Geometry check sheet. Reference: the model listing, model coordinates, mm. A direction names the side the tool comes from. Round coordinates to 2 decimals unless told otherwise and drop trailing zeros. Loops run counter-clockwise (first coordinate to the right, second up) from the corner with the lowest first, then second, coordinate; pieces in that order, holes last. Notation, with made-up numbers: (77.25, 34.25) -> (96.25, 34.25) arc R19 ccw to (96.25, 58.25) -> close; hole circle Ø4 at (-38, 28). An arc over 180 degrees is marked (long way). Use a Markdown table: item, result. Add a question column.
Q1. Release check for a two-part mould opening along Y. For faces 1 (the face through (46.297, -31.359, 14.79)), 2 (the face through (47.5, 0, 15)), 3 (the face through (-46.297, 31.359, 14.79)), 4 (the face through (23.856, -5.745, 28.986)) record: released by +Y, released by -Y, zero draft, split by the parting line, or undercut.
Q2. Gauge pin test, flat end, axial feed: P1, Ø9, axis at x = 2.5, y = -6, coming from the +Z side. Record the tip position at first contact, or that the pin passes through.
Q3. Sectioned sample at A-A, the plane x = 10. Enter the section's corners in (y, z).
Q4. Set-up check for faces 5 (the face through (46.359, 31.297, 14.79)), 6 (the face through (10, 0, 28)): record each of +Z, -Z, +X, -X, +Y, -Y from which the full face is reachable in a straight line by a thin tool's end or side.
Q5. Sectioned sample at B-B, the plane y = 0. Enter the section's corners in (x, z).
Q6. Material ranges on L1, parallel to Y at x = 10, z = 28.7, recorded low to high.
```python
from build123d import *

# Parameters (mm, degrees)
ENVOLVENTE_95X65X30_DEPTH = 30
VENTILADOR_START          = 28
CROQUIS2_R                = 15
VENTILADOR_DEPTH          = 2


with BuildPart() as part:
    # Croquis1 → Envolvente_95x65x30 (new body)
    with BuildSketch(Plane.XY):
        with BuildLine():
            Line((-43.5, -32.5), (43.5, -32.5))
            ThreePointArc((43.5, -32.5), (46.328427125, -31.328427125), (47.5, -28.5))
            Line((47.5, -28.5), (47.5, 28.5))
            ThreePointArc((47.5, 28.5), (46.328427125, 31.328427125), (43.5, 32.5))
            Line((43.5, 32.5), (-43.5, 32.5))
            ThreePointArc((-43.5, 32.5), (-46.328427125, 31.328427125), (-47.5, 28.5))
            Line((-47.5, 28.5), (-47.5, -28.5))
            ThreePointArc((-47.5, -28.5), (-46.328427125, -31.328427125), (-43.5, -32.5))
        make_face()
    extrude(amount=ENVOLVENTE_95X65X30_DEPTH)

    # Croquis2 → Ventilador (cut)
    with BuildSketch(Plane.XY.offset(VENTILADOR_START)):
        with Locations((10, 0)):
            Circle(CROQUIS2_R)
    extrude(amount=VENTILADOR_DEPTH, mode=Mode.SUBTRACT)


solid = part.part
```
Values:
| question | item | result |
|---|---|---|
| 1 | face 1 | released by -Y |
| 1 | face 2 | zero draft |
| 1 | face 3 | released by +Y |
| 1 | face 4 | undercut |
| 2 | P1 | z = 28 |
| 3 | outline | (-32.5, 0) -> (32.5, 0) -> (32.5, 30) -> (15, 30) -> (15, 28) -> (-15, 28) -> (-15, 30) -> (-32.5, 30) -> close |
| 4 | face 5 | +Z, -Z, +X, +Y |
| 4 | face 6 | +Z |
| 5 | outline | (-47.5, 0) -> (47.5, 0) -> (47.5, 30) -> (25, 30) -> (25, 28) -> (-5, 28) -> (-5, 30) -> (-47.5, 30) -> close |
| 6 | L1 | -32.5 to -15, 15 to 32.5 |
